For this review, take the finished solid that the model builds, in its own axes (mm). A direction names the side the tool comes from. Give positions to 0.01 mm unless a question says otherwise; leave off trailing zeros. Order: outer loops, then holes, each group sorted by start corner. A loop starts at its lowest first (then second) coordinate and runs counter-clockwise, first axis right, second up.
from build123d import *

# Parameters (mm, degrees)
F0_W     = 60
F0_H     = 60
F1_DEPTH = 5
F2_R     = 25
F3_DEPTH = 2
F4_R     = 10
F5_W     = 3
F5_H     = 6
F5_W_2   = 6
F5_H_2   = 3
F6_DEPTH = 1


with BuildPart() as f1:
    # F0 (on Top) → F1 (new body)
    with BuildSketch(Plane.XY):
        Rectangle(F0_W, F0_H)
    extrude(amount=F1_DEPTH)

    # F2 (on face) → F3 (cut)
    with BuildSketch(Plane.XY.offset(5)):
        Circle(F2_R)
    extrude(amount=-F3_DEPTH, mode=Mode.SUBTRACT)

    # F4
    f4_edges = [f1.edges().sort_by_distance(p)[0] for p in [
        (-30, -30, 2.5),
        (30, -30, 2.5),
        (30, 30, 2.5),
        (-30, 30, 2.5),
    ]]
    fillet(f4_edges, radius=F4_R)

    # F5 (on face) → F6 (cut)
    with BuildSketch(Plane.XY.offset(3)):
        with Locations((0, 16)):
            Rectangle(F5_W, F5_H)
        with Locations((-16, 0)):
            Rectangle(F5_W_2, F5_H_2)
        with Locations((0, -16)):
            Rectangle(F5_W, F5_H)
        with Locations((16, 0)):
            Rectangle(F5_W_2, F5_H_2)
    extrude(amount=-F6_DEPTH, mode=Mode.SUBTRACT)


solid = f1.part
1) We need section C-C on x = 7. Give the boundary of the cut face in (y, z).
Answer sheet:
outline: (-30, 0) - (30, 0) - (30, 5) - (24, 5) - (24, 3) - (-24, 3) - (-24, 5) - (-30, 5) - close
2) We need section A-A on y = 0. Give the boundary of the cut face in (x, z), then the cut area to 3 significant figures.
Answer sheet:
outline: (-30, 0) - (30, 0) - (30, 5) - (25, 5) - (25, 3) - (19, 3) - (19, 2) - (13, 2) - (13, 3) - (-13, 3) - (-13, 2) - (-19, 2) - (-19, 3) - (-25, 3) - (-25, 5) - (-30, 5) - close
area: 188 mm2
3) Tool access review of faces 5 (the face through (-16, 0, 2)), 6 (the face through (26.99, -27.15, 2.54)): name each direction out of +Z, -Z, +X, -X, +Y, -Y from which nothing blocks a thin tool from reaching the whole face with its end or side.
Answer sheet:
face 5: +Z
face 6: +Z, -Z, +X, -Y
4) Draft analysis for pull direction Y (two halves, no side actions). For faces 1 (the face through (30, 0, 2)), 2 (the face through (23.846, 7.509, 4.014)), 3 (the face through (26.99, 27.15, 2.54)), 4 (the face through (0, -16, 2)), state which applies: +Y half, -Y half, draft (parallel to the pull), parting line (faces both ways), or undercut.
Answer sheet:
face 1: draft
face 2: undercut
face 3: +Y half
face 4: undercut
5) Clearance check with a flat-ended pin moving along its axis: pin 1 (3.5 mm diameter, centred on x = -17, y = -0.5, fed in from +Z). State where the tip first meets the part, or that it passes through.
Answer sheet:
pin 1: stops at z = 3
6) To check wall thickness, follow line 1 (Y direction, x = 0, z = 3.7); line 2 (Y direction, x = 14, z = 2.65); line 3 (Z direction, x = 3, y = -19). State the ranges of each line that lie inside material, in increasing order.
Answer sheet:
line 1: y = -30 to -25, 25 to 30
line 2: y = -30 to -1.5, 1.5 to 30
line 3: z = 0 to 3
7) We need section D-D on x = 15. Give the boundary of the cut face in (y, z).
Answer sheet:
outline: (-30, 0) - (30, 0) - (30, 5) - (20, 5) - (20, 3) - (1.5, 3) - (1.5, 2) - (-1.5, 2) - (-1.5, 3) - (-20, 3) - (-20, 5) - (-30, 5) - close
